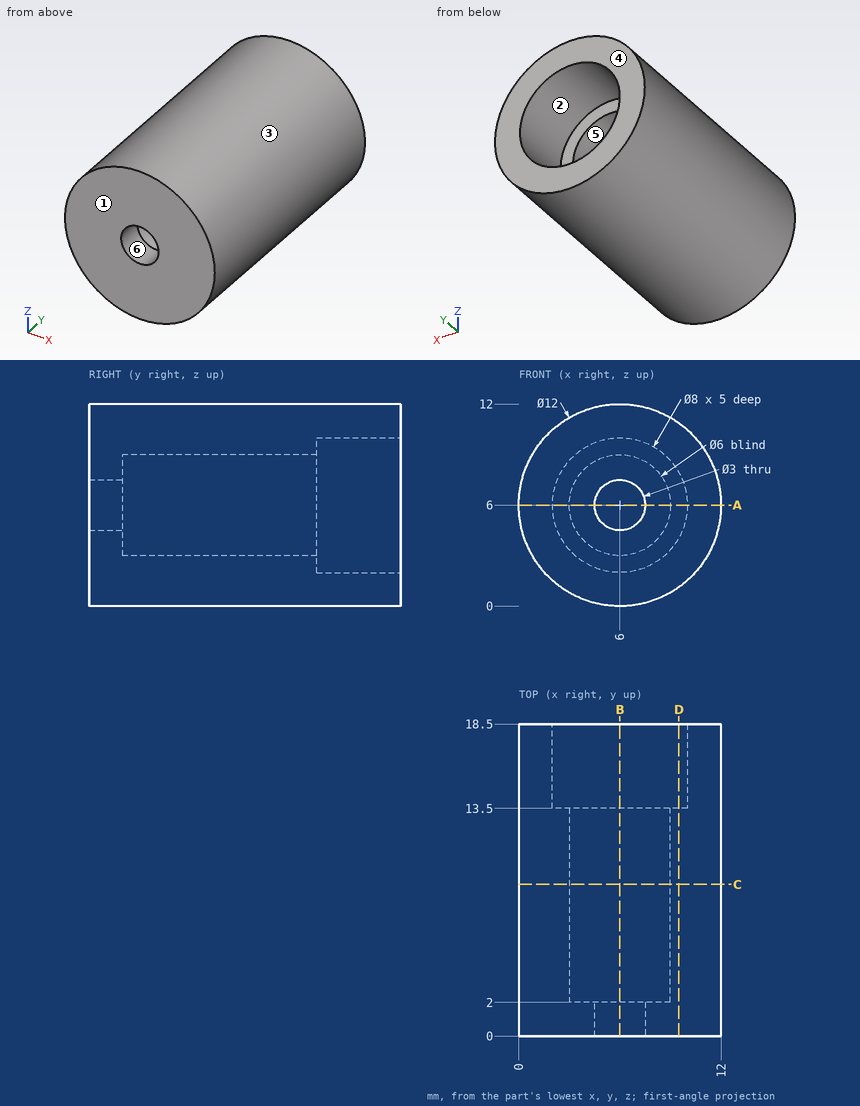
Can you work these out from the drawing? Everything is in mm from the part's minimum corner. A direction names the side the tool comes from. Give positions to 0.01 mm unless a question says otherwise; leave off trailing zeros. Order: outer loops, then holes, each group sorted by start corner. A loop starts at its lowest first (then second) coordinate and runs counter-clockwise, first axis right, second up. Notation, with made-up numbers: M 89.25,25.25 L 122.25,25.25 A16 cw 122.25,38.25 Z; hole C 50.5,-6.75 d11. An arc over 180 degrees is marked long. Use a Markdown table: item, result. Add a question column.
Item 1: For the marked faces 1 and 2, which set-ups out of +Z, -Z, +X, -X, +Y, -Y let a thin tool reach every point of the face, with its end or its side?
Item 2: Suppose I cut it at D-D (x = 9.5). List the corners of the cut face in (y, z) for me, then the cut area to 3 significant figures.
Item 3: If I drill on L1, parallel to Z at x = 6, y = 1.1; L2, parallel to X at y = 9.5, z = 6, over which ranges is the centre line in solid material (lowest first)? Write a range as [from, to].
Item 4: Suppose I cut it at C-C (y = 9). List the corners of the cut face in (x, z) for me, then the cut area to 3 significant figures.
Item 5: Suppose I cut it at A-A (z = 6). List the corners of the cut face in (x, y) for me, then the cut area to 3 significant figures.
Item 6: We'd pull the mould along X, two halves only. Please class the marked faces 3, 4, 5 and 6: +X half, -X half, draft (parallel to the pull), parting line (faces both ways), or undercut.
Item 7: Will these pins go through, and if not, where does the flat tip stop? pin 1 (5 mm diameter, centred on x = 6, z = 6, fed in from -Y); pin 2 (4 mm diameter, centred on y = 9, z = 9.5, fed in from -X); pin 3 (1.5 mm diameter, centred on y = 15.5, z = 9.5, fed in from -X); pin 4 (1 mm diameter, centred on y = 14.5, z = 5, fed in from +X).
Item 8: Suppose I cut it at B-B (x = 6). List the corners of the cut face in (y, z) for me.
Answer sheet:
| question | item | result |
|---|---|---|
| 1 | face 1 | +Z, -Z, +X, -X, -Y |
| 1 | face 2 | +Y |
| 2 | outline | M 0,1.13 L 18.5,1.13 L 18.5,4.06 L 13.5,4.06 L 13.5,7.94 L 18.5,7.94 L 18.5,10.87 L 0,10.87 Z |
| 2 | area | 161 mm² |
| 3 | L1 | z = [0, 4.5], [7.5, 12] |
| 3 | L2 | x = [0, 3], [9, 12] |
| 4 | outline | C 6,6 d12; hole C 6,6 d6 |
| 4 | area | 84.8 mm² |
| 5 | outline | M 0,0 L 4.5,0 L 4.5,2 L 3,2 L 3,13.5 L 2,13.5 L 2,18.5 L 0,18.5 Z; M 7.5,0 L 12,0 L 12,18.5 L 10,18.5 L 10,13.5 L 9,13.5 L 9,2 L 7.5,2 Z |
| 5 | area | 107 mm² |
| 6 | face 3 | parting line |
| 6 | face 4 | draft |
| 6 | face 5 | undercut |
| 6 | face 6 | undercut |
| 7 | pin 1 | stops at y = 0 |
| 7 | pin 2 | stops at x = 0.19 |
| 7 | pin 3 | stops at x = 0.67 |
| 7 | pin 4 | stops at x = 11.98 |
| 8 | outline | M 0,0 L 18.5,0 L 18.5,2 L 13.5,2 L 13.5,3 L 2,3 L 2,4.5 L 0,4.5 Z; M 0,7.5 L 2,7.5 L 2,9 L 13.5,9 L 13.5,10 L 18.5,10 L 18.5,12 L 0,12 Z |
